from build123d import *

# Parameters (mm, degrees)
ESQUISSE1_W     = 40
ESQUISSE1_H     = 10
CHANFREIN1_SIZE = 2


with BuildPart() as part:
    # Esquisse1 → Révolution1 (revolve)
    with BuildSketch(Plane.XY):
        with Locations((-20, 35)):
            Rectangle(ESQUISSE1_W, ESQUISSE1_H)
        Polygon((0, 40), (0, 30), (20, 30), (20, 60), (0, 60), align=None)
    revolve(axis=Axis((0, 0, 0), (-1, 0, 0)))

    # Chanfrein1
    chanfrein1_edges = [part.edges().sort_by_distance(p)[0] for p in [
        (-40, -40, 0),
        (20, -30, 0),
        (-40, -30, 0),
    ]]
    chamfer(chanfrein1_edges, length=CHANFREIN1_SIZE)


solid = part.part
The listing builds one solid part. Answer for the finished solid, in the listing's coordinates (mm). A direction names the side the tool comes from. Coordinates: 2 decimals unless noted, no trailing zeros. Loops run counter-clockwise (first coordinate to the right, second up) from the corner with the lowest first, then second, coordinate; pieces in that order, holes last. Notation, with made-up numbers: (88.25, 47.5) -> (116.25, 47.5) arc R29 ccw to (116.25, 79.5) -> close; hole circle Ø5 at (6.5, 78). An arc over 180 degrees is marked (long way). Write item = value, one per line. Start each with the question number.
1) A cutting plane is placed at C-C (x = -6.5). Give the vertices of the cut face in (y, z), then the cut area to 3 significant figures.
2) A cutting plane is placed at A-A (y = 0). Give the vertices of the cut face in (x, z), then the cut area to 3 significant figures.
3) The mould has two halves that part along Z. Classify faces 1 (the face through (0, 12, 39)), 2 (the face through (-9.61, -29.97, -1.32)), 3 (the face through (18.13, 13.9, 26.73)), 4 (the face through (-39.875, -8.265, 37.219)): released by +Z, released by -Z, zero draft, split by the parting line, or undercut.
4) Straight lines are drawn through the part: line 1 (Y direction, x = -1, z = 0); line 2 (Y direction, x = 7, z = 0). For each, find the intervals that lie inside material, in ascending order. Write a range as from..to.
5) Given pin 1 Ø4 at (x, z) = (-21.5, 14) entering from -Y; pin 2 Ø6 at (x, z) = (-23.5, -38.5) entering from +Y; pin 3 Ø6 at (x, y) = (-32, 8) entering from +Z, each flat-ended and moving along its own axis, determine where each tip first touches the part or whether it passes through.
6) A cutting plane is placed at D-D (y = -48). Give the vertices of the cut face in (x, z).
7) A tool of negligible diameter and unlimited length cuts with its end or side. For faces 5 (the face through (-18.73, -8.67, 39.05)), 6 (the face through (-40, 17, 28)), from which of +Z, -Z, +X, -X, +Y, -Y can it reach the whole face along a straight path? Write none if from no direction.
Responses:
q1.outline = circle Ø80 at (0, 0); hole circle Ø60 at (0, 0)
q1.area = 2,200 mm²
q2.outline = (-40, -38) -> (-38, -40) -> (0, -40) -> (0, -60) -> (20, -60) -> (20, -32) -> (18, -30) -> (-38, -30) -> (-40, -32) -> close; (-40, 32) -> (-38, 30) -> (18, 30) -> (20, 32) -> (20, 60) -> (0, 60) -> (0, 40) -> (-38, 40) -> (-40, 38) -> close
q2.area = 1,990 mm²
q3.face_1 = zero draft
q3.face_2 = undercut
q3.face_3 = undercut
q3.face_4 = split by the parting line
q4.line_1 = -40..-30, 30..40
q4.line_2 = -60..-30, 30..60
q5.pin_1 = -38.16
q5.pin_2 = 18.43
q5.pin_3 = 39.69
q6.outline = (0, -36) -> (20, -36) -> (20, 36) -> (0, 36) -> close
q7.face_5 = -X
q7.face_6 = +Z, -Z, -X, +Y, -Y
